Build history of the part. All positions in model axes, mm. A direction names the side the tool comes from. Round coordinates to 2 decimals unless told otherwise and drop trailing zeros. Loops run counter-clockwise (first coordinate to the right, second up) from the corner with the lowest first, then second, coordinate; pieces in that order, holes last.
from build123d import *

# Parameters (mm, degrees)
SKETCH1_W           = 82.2
SKETCH1_H           = 3.6
BOSS_EXTRUDE1_DEPTH = 82.2
SKETCH2_W           = 76.4
SKETCH2_H           = 76.4
CUT_EXTRUDE1_DEPTH  = 1.31
SKETCH4_R           = 1
CUT_EXTRUDE3_DEPTH  = 1.31
SKETCH3_W           = 46
SKETCH3_H           = 46
CUT_EXTRUDE2_DEPTH  = 92.930920261


with BuildPart() as part:
    # Sketch1 → Boss-Extrude1 (new body)
    with BuildSketch(Plane(origin=(0, 0, 0), x_dir=(1, 0, 0), z_dir=(0, 1, 0))):
        with Locations((0, 1.8)):
            Rectangle(SKETCH1_W, SKETCH1_H)
    extrude(amount=BOSS_EXTRUDE1_DEPTH)

    # Sketch2 → Cut-Extrude1 (cut)
    with BuildSketch(Plane(origin=(0, 0, -3.6), x_dir=(-1, 0, 0), z_dir=(0, 0, -1))):
        with Locations((0, 41.1)):
            Rectangle(SKETCH2_W, SKETCH2_H)
    extrude(amount=-CUT_EXTRUDE1_DEPTH, mode=Mode.SUBTRACT)

    # Sketch4 → Cut-Extrude3 (cut)
    with BuildSketch(Plane(origin=(0, 0, -3.6), x_dir=(-1, 0, 0), z_dir=(0, 0, -1))):
        with Locations((38.2, 2.9)):
            Circle(SKETCH4_R)
        with Locations((38.2, 79.3)):
            Circle(SKETCH4_R)
        with Locations((-38.2, 2.9)):
            Circle(SKETCH4_R)
        with Locations((-38.2, 79.3)):
            Circle(SKETCH4_R)
    extrude(amount=-CUT_EXTRUDE3_DEPTH, mode=Mode.SUBTRACT)

    # Sketch3 → Cut-Extrude2 (cut, through all)
    with BuildSketch(Plane(origin=(0, 0, -2.29), x_dir=(-1, 0, 0), z_dir=(0, 0, -1))):
        with Locations((0, 41.1)):
            Rectangle(SKETCH3_W, SKETCH3_H)
    extrude(amount=-CUT_EXTRUDE2_DEPTH, mode=Mode.SUBTRACT)


solid = part.part
(1) Slice it at B-B on x = 17. List the corners of the cut face in (y, z).
Responses:
outline: (0, -3.6) - (2.9, -3.6) - (2.9, -2.29) - (18.1, -2.29) - (18.1, 0) - (0, 0) - close; (64.1, -2.29) - (79.3, -2.29) - (79.3, -3.6) - (82.2, -3.6) - (82.2, 0) - (64.1, 0) - close
(2) Probe line 1 (Y direction, x = -12, z = -2.6); line 2 (X direction, y = 19, z = -0.9); line 3 (Y direction, x = 10, z = -2.15). List the from-to ranges inside material, lowest first.
Responses:
line 1: y = 0 to 2.9, 79.3 to 82.2
line 2: x = -41.1 to -23, 23 to 41.1
line 3: y = 0 to 18.1, 64.1 to 82.2
(3) Slice it at A-A on y = 38. List the corners of the cut face in (x, z), plus the area to 3 significant figures.
Responses:
outline: (-41.1, -3.6) - (-38.2, -3.6) - (-38.2, -2.29) - (-23, -2.29) - (-23, 0) - (-41.1, 0) - close; (23, -2.29) - (38.2, -2.29) - (38.2, -3.6) - (41.1, -3.6) - (41.1, 0) - (23, 0) - close
area: 90.5 mm2
(4) Pull direction Y, two halves, no side cores. Call faces 1 (the face through (-1, 0, -2)), 2 (the face through (-1, 82.2, -2)), 3 (the face through (-38.93, 79.983, -2.954)), 4 (the face through (0, 18.1, -1)): +Y half, -Y half, draft (parallel to the pull), parting line (faces both ways), or undercut.
Responses:
face 1: -Y half
face 2: +Y half
face 3: undercut
face 4: undercut
(5) Slice it at D-D on x = 32. List the corners of the cut face in (y, z).
Responses:
outline: (0, -3.6) - (2.9, -3.6) - (2.9, -2.29) - (79.3, -2.29) - (79.3, -3.6) - (82.2, -3.6) - (82.2, 0) - (0, 0) - close
(6) Slice it at C-C on z = -0.85. List the corners of the cut face in (x, y), plus the area to 3 significant figures.
Responses:
outline: (-41.1, 0) - (41.1, 0) - (41.1, 82.2) - (-41.1, 82.2) - close; hole (-23, 18.1) - (23, 18.1) - (23, 64.1) - (-23, 64.1) - close
area: 4,640 mm2
(7) Pin check, flat tip, straight feed: P1, Ø1.2, axis at x = -38.2, y = 79.3, coming from the -Z side. Stop position of the tip, or through.
Responses:
P1: stops at z = -2.29
(8) Which spindle directions (+Z, -Z, +X, -X, +Y, -Y) get a long thin tool onto all of the face, cutting with end or side? Do faces 5 (the face through (41.1, 41, -2)), 6 (the face through (38.93, 2.217, -2.954)), 7 (the face through (-23, 41, -1)). Say none if no direction does.
Responses:
face 5: +Z, -Z, +X, +Y, -Y
face 6: -Z
face 7: +Z, -Z
